The model under review builds one solid part; all positions refer to its coordinate system, in mm. Coordinates: 2 decimals unless noted, no trailing zeros. Loops run counter-clockwise (first coordinate to the right, second up) from the corner with the lowest first, then second, coordinate; pieces in that order, holes last. Notation, with made-up numbers: M 36,1 L 86,1 A14 ccw 86,12 Z; hole C 22,-12.75 d11. An arc over 180 degrees is marked long. One line per item, written item: value.
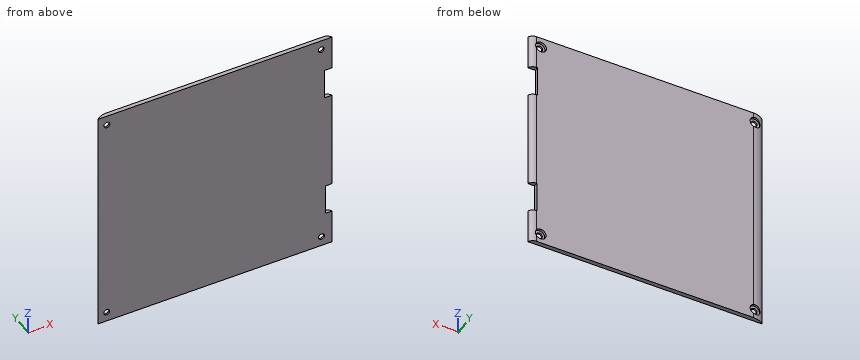
```python
from build123d import *

# Parameters (mm, degrees)
SKETCH1_W                                   = 142
SKETCH1_H                                   = 140
BOSS_EXTRUDE1_DEPTH                         = 2.5
SKETCH6_W                                   = 4
SKETCH6_H                                   = 18.75
CUT_EXTRUDE1_DEPTH                          = 100.735901259
SKETCH7_W                                   = 4.5
SKETCH7_H                                   = 18.75
CUT_EXTRUDE2_DEPTH                          = 100.735901259
CBORE_FOR_M3_CHEESE_HEAD_SCREW1_D           = 3.6
CBORE_FOR_M3_CHEESE_HEAD_SCREW1_CBORE_D     = 6.5
CBORE_FOR_M3_CHEESE_HEAD_SCREW1_CBORE_DEPTH = 1.5
FILLET4_R                                   = 10
FILLET7_R                                   = 4


with BuildPart() as part:
    # Sketch1 → Boss-Extrude1 (new body)
    with BuildSketch(Plane(origin=(0, 0, 0), x_dir=(1, 0, 0), z_dir=(0, 1, 0))):
        Rectangle(SKETCH1_W, SKETCH1_H)
    extrude(amount=-BOSS_EXTRUDE1_DEPTH)

    # Sketch6 → Cut-Extrude1 (cut, through all)
    with BuildSketch(Plane(origin=(0, 0, 0), x_dir=(1, 0, 0), z_dir=(0, 1, 0))):
        with Locations((69, 39.625)):
            Rectangle(SKETCH6_W, SKETCH6_H)
    extrude(amount=-CUT_EXTRUDE1_DEPTH, mode=Mode.SUBTRACT)

    # Sketch7 → Cut-Extrude2 (cut, through all)
    with BuildSketch(Plane(origin=(0, 0, 0), x_dir=(1, 0, 0), z_dir=(0, 1, 0))):
        with Locations((68.75, -39.625)):
            Rectangle(SKETCH7_W, SKETCH7_H)
    extrude(amount=-CUT_EXTRUDE2_DEPTH, mode=Mode.SUBTRACT)

    # CBORE for M3 Cheese Head Screw1 (through all)
    with Locations(Plane(origin=(-65.6357603, 0, -64), x_dir=(0, 0, 1), z_dir=(0, 1, 0))):
        with Locations((0, 0), (0, 130.23152632), (128, 130.05051113), (128, 0.0399943)):
            CounterBoreHole(CBORE_FOR_M3_CHEESE_HEAD_SCREW1_D / 2, CBORE_FOR_M3_CHEESE_HEAD_SCREW1_CBORE_D / 2, CBORE_FOR_M3_CHEESE_HEAD_SCREW1_CBORE_DEPTH)

    # Fillet4
    # the kernel refuses this fillet: 10 mm, written as the material it takes off along each edge
    with BuildSketch(Plane(origin=(-71, 0, 86.535945694), x_dir=(0, -1, 0), z_dir=(0, 0, -1))) as fillet4_piece_1:
        with BuildLine():
            CenterArc((10, -6.614378278), FILLET4_R, 138.590377891, 41.409622109)
            Line((0, -6.614378278), (-0.2, -6.614378278))
            Line((-0.2, -6.614378278), (-0.2, 0))
            Line((-0.2, 0), (0, 0.2))
            ThreePointArc((0, 0.2), (1.25, 0.2), (2.35, 0.132287566))
            Line((2.35, 0.132287566), (2.5, 0))
        make_face()
    extrude(amount=173.071891388, mode=Mode.SUBTRACT)

    # Fillet7
    # the kernel refuses this fillet: 4 mm, written as the material it takes off along each edge
    with BuildSketch(Plane(origin=(71, 0, 39.729751891), x_dir=(-1, 0, 0), z_dir=(0, 0, 1)), Plane(origin=(71, 0, -79.270248109), x_dir=(-1, 0, 0), z_dir=(0, 0, 1))) as fillet7_piece_1:
        with BuildLine():
            CenterArc((3.708099244, 4), FILLET7_R, 202.024312837, 67.975687163)
            Line((0, 2.5), (-0.074161985, 2.47))
            ThreePointArc((-0.074161985, 2.47), (-0.08, 1.25), (-0.08, 0))
            Line((-0.08, 0), (0, -0.08))
            Line((0, -0.08), (3.708099244, -0.08))
            Line((3.708099244, -0.08), (3.708099244, 0))
        make_face()
    extrude(amount=39.540496218, mode=Mode.SUBTRACT)
    with BuildSketch(Plane(origin=(71, 0, -39.520248109), x_dir=(-1, 0, 0), z_dir=(0, 0, 1))) as fillet7_piece_2:
        with BuildLine():
            CenterArc((3.708099244, 4), FILLET7_R, 202.024312837, 67.975687163)
            Line((0, 2.5), (-0.074161985, 2.47))
            ThreePointArc((-0.074161985, 2.47), (-0.08, 1.25), (-0.08, 0))
            Line((-0.08, 0), (0, -0.08))
            Line((0, -0.08), (3.708099244, -0.08))
            Line((3.708099244, -0.08), (3.708099244, 0))
        make_face()
    extrude(amount=79.040496218, mode=Mode.SUBTRACT)


solid = part.part
```
(1) Insertion check: pin 1 Ø2 at (x, z) = (64.41, 64) entering from +Y; pin 2 Ø2 at (x, z) = (-64.5, -63) entering from +Y; pin 3 Ø0.8 at (y, z) = (-1.5, 40.5) entering from +X. Each pin has a flat end and moves straight along its axis. Give the tip position at first contact, or say it passes through.
Checks:
pin 1: through
pin 2: y = -1.5
pin 3: x = 66.5
(2) To check wall thickness, follow L1, parallel to Z at x = 64.5, y = -1; L2, parallel to X at y = -2, z = 64; L3, parallel to X at y = -1.7, z = 64. State the ranges of each line that lie inside material, in increasing order. Write a range as [from, to].
Checks:
L1: [-70, -67.25], [-60.75, 60.75], [67.25, 70]
L2: [-70.39, -67.4], [-63.8, 62.61], [66.21, 70.76]
L3: [-69.96, -67.4], [-63.8, 62.61], [66.21, 70.56]
(3) Add section C-C on z = 34.5. State the section outline as (x, y) points, then the cut area to 3 significant figures.
Checks:
outline: M -71,-2.5 L 66.5,-2.5 L 66.5,0 L -64.39,0 A10 ccw Z
area: 339 mm^2
(4) Add section B-B on y = -0.5. State the section outline as (x, z) points, then the cut area to 3 significant figures.
Checks:
outline: M -67.51,-70 L 69.23,-70 L 69.23,-49 L 67,-49 L 67,-30.25 L 69.23,-30.25 L 69.23,30.25 L 66.5,30.25 L 66.5,49 L 69.23,49 L 69.23,70 L -67.51,70 L -67.51,66.63 A3.25 cw long -67.51,61.37 L -67.51,-61.34 A3.25 cw long -67.51,-66.66 Z; hole C 64.41,64 d6.5; hole C 64.6,-64 d6.5
area: 18,900 mm^2
(5) Add section D-D on z = -9.5. State the section outline as (x, y) points, then the cut area to 3 significant figures.
Checks:
outline: M -71,-2.5 L 71,-2.5 A4 ccw 67.29,0 L -64.39,0 A10 ccw Z
area: 347 mm^2
(6) Add section A-A on z = -64. State the section outline as (x, y) points.
Checks:
outline: M -71,-2.5 L -67.44,-2.5 L -67.44,-1.5 L -68.89,-1.5 L -68.89,-1.07 A10 ccw Z; M -63.84,-2.5 L 62.8,-2.5 L 62.8,-1.5 L 61.35,-1.5 L 61.35,0 L -62.39,0 L -62.39,-1.5 L -63.84,-1.5 Z; M 66.4,-2.5 L 71,-2.5 A4 ccw 67.85,-0.04 L 67.85,-1.5 L 66.4,-1.5 Z
